Read the model definition and answer for the solid it produces. Units are mm, in the model's axes. A direction names the side the tool comes from. Round coordinates to 2 decimals unless told otherwise and drop trailing zeros. Write each loop counter-clockwise with the first axis right and the second up, starting at its lowest first coordinate (ties: lowest second). Pieces come first, ordered by that corner, then holes. Notation, with made-up numbers: (-31, 76) - (-7, 76) arc R25 ccw to (-7, 113) - close; hole circle Ø10 at (42, 49.5). An arc over 180 degrees is marked (long way). Answer as CSV lines item,"result". Start each with the question number.
1) Find section A-A on x = 0. Determine the outline of the cut face in (y, z).
2) For a pull along X with two mould halves and no side action, classify faces 3 (the flat face through (0, 0, 0)), 4 (the cylindrical face through (-0.07, -1.5, -2.32)), 5 (the flat face through (0, 1, -5)) as +X half, -X half, draft (parallel to the pull), parting line (faces both ways), or undercut.
3) Which of the six approach directions +Z, -Z, +X, -X, +Y, -Y give full straight-line access (tool end or side, diameter ignored) to faces 1 (the flat face through (-0.87, -0.49, -5.41)), 2 (the conical face through (-2, 0, -5))?
4) Each of these flat-tipped pins is pushed along its axis until it touches: pin 1 (0.9 mm diameter, centred on x = 0, z = -5.5, fed in from +Y); pin 2 (1.5 mm diameter, centred on x = 0.5, z = -3.5, fed in from +Y). Where does it stop, or does it pass through?
5) Consider line 1 along Z through (x, y) = (-0.25, 0.85); line 2 along Y through (x, z) = (1.1, -5.35); line 3 along Y through (x, z) = (-0.7, -5.45). Determine where each line is inside the solid, lowest interval first.
6) Find section B-B on z = -0.55. Determine the outline of the cut face in (x, y).
Autodesk Inventor part; units mm, degrees
ref_plane "YZ Plane" through (0, 0, 0) normal (1, 0, 0) x (0, 1, 0)
ref_plane "XZ Plane" through (0, 0, 0) normal (0, 1, 0) x (-1, 0, 0)
ref_plane "XY Plane" through (0, 0, 0) normal (0, 0, 1) x (1, 0, 0)
sketch "Sketch4" plane through (0, 0, 0) normal (1, 0, 0) x (0, 1, 0)
  line L0 (0, 0) -> (0, -6)
  line L1 (0, -6) -> (3, -6)
  line L2 (3, -6) -> (1.5, -4.5)
  line L3 (1.5, -4.5) -> (1.5, 0)
  line L4 (1.5, 0) -> (0, 0)
  dimension "d11" = 6
  dimension "d12" = 3
  dimension "d15" = 6
  dimension "d16" = 45
revolve "Revolution1" add sketch "Sketch4" angle 360 about axis through (0, 0, 0) along (0, 0, -1)
sketch "Sketch5" plane through (0, 0, -6) normal (0, 0, -1) x (-1, 0, 0)
  line L0 (1.1547, 0) -> (0.5774, -1)
  line L1 (0.5774, -1) -> (-0.5774, -1)
  line L2 (-0.5774, -1) -> (-1.1547, 0)
  line L3 (-1.1547, 0) -> (-0.5774, 1)
  line L4 (-0.5774, 1) -> (0.5774, 1)
  line L5 (0.5774, 1) -> (1.1547, 0)
  point P0 (0, 0)
  point P1 (0, 0)
  dimension "d18" = 2
extrude "Extrusion5" cut sketch "Sketch5" against normal blind 1.2
chamfer "Chamfer2" distance 0.2 angle 45 1 edges at (0, -1.5, 0)
thread "Thread1"
properties part number "M3 x 6 mm FHCS" material "Stainless Steel"
Check values:
1,outline,"(-3, -6) - (-1, -6) - (-1, -4.8) - (1, -4.8) - (1, -6) - (3, -6) - (1.5, -4.5) - (1.5, -0.2) - (1.3, 0) - (-1.3, 0) - (-1.5, -0.2) - (-1.5, -4.5) - close"
2,face 3,"draft"
2,face 4,"parting line"
2,face 5,"undercut"
3,face 1,"-Z"
3,face 2,"+Z"
4,pin 1,"stops at y = 2.95"
4,pin 2,"stops at y = 1.5"
5,line 1,"z = -4.8 to 0"
5,line 2,"y = -2.08 to -0.09, 0.09 to 2.08"
5,line 3,"y = -2.35 to -0.79, 0.79 to 2.35"
6,outline,"circle Ø3 at (0, 0)"
